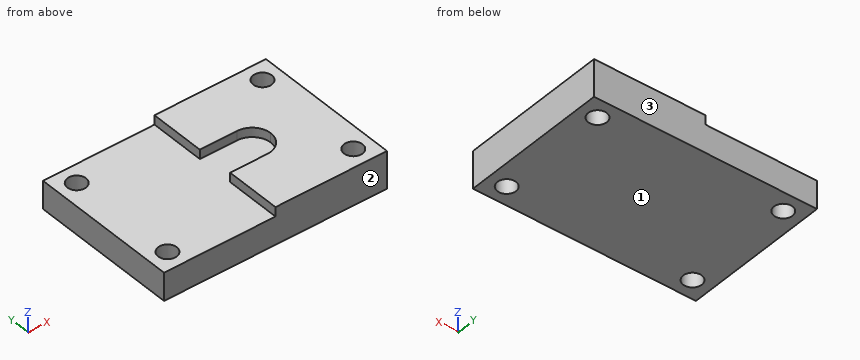
```python
from build123d import *

# Parameters (mm, degrees)
F0_W     = 76.2
F0_H     = 50.8
F1_DEPTH = 12.7
F2_R     = 3.175
F3_DEPTH = 12.701
F5_DEPTH = 3.175
F6_W     = 38.1
F6_H     = 50.8
F7_DEPTH = 3.175


with BuildPart() as f1:
    # F0 (on Top) → F1 (new body)
    with BuildSketch(Plane.XY):
        Rectangle(F0_W, F0_H)
    extrude(amount=F1_DEPTH)

    # F2 (on face) → F3 (cut, through all)
    with BuildSketch(Plane.XY.offset(12.7)):
        with Locations((-31.75, 19.05)):
            Circle(F2_R)
        with Locations((31.75, 19.05)):
            Circle(F2_R)
        with Locations((31.75, -19.05)):
            Circle(F2_R)
        with Locations((-31.75, -19.05)):
            Circle(F2_R)
    extrude(amount=-F3_DEPTH, mode=Mode.SUBTRACT)

    # F4 (on face) → F5 (cut)
    with BuildSketch(Plane.XY.offset(12.7)):
        with BuildLine():
            Line((-12.7, -6.35), (12.7, -6.35))
            ThreePointArc((12.7, -6.35), (17.190128, -4.490128), (19.05, 0))
            ThreePointArc((19.05, 0), (17.190128, 4.490128), (12.7, 6.35))
            Line((12.7, 6.35), (-12.7, 6.35))
            ThreePointArc((-12.7, 6.35), (-17.190128, 4.490128), (-19.05, 0))
            ThreePointArc((-19.05, 0), (-17.190128, -4.490128), (-12.7, -6.35))
        make_face()
    extrude(amount=-F5_DEPTH, mode=Mode.SUBTRACT)

    # F6 (on face) → F7 (cut, through all)
    with BuildSketch(Plane.XY.offset(12.7)):
        with Locations((-19.05, 0)):
            Rectangle(F6_W, F6_H)
    extrude(amount=-F7_DEPTH, mode=Mode.SUBTRACT)


solid = f1.part
```
Build history of the part. All positions in model axes, mm. Face numbers are marked on the shaded views. Give positions to 0.01 mm unless a question says otherwise; leave off trailing zeros. Loops run counter-clockwise (first coordinate to the right, second up) from the corner with the lowest first, then second, coordinate; pieces in that order, holes last. Notation, with made-up numbers: (-34, 61.5) -> (-13, 61.5) arc R7 ccw to (-13, 68.5) -> close; hole circle Ø9 at (78, 54). An arc over 180 degrees is marked (long way). One line per question, with ' | ' between items. Start each with the question number.
1) Cut at C-C (z = 4). Give the cut face in (x, y) (3 decimals), plus the area to 3 significant figures.
2) Pin check, flat tips, straight feed: pin 1 (2.5 mm diameter, centred on y = 17, z = 11.5, fed in from -X); pin 2 (4 mm diameter, centred on x = 31.75, y = -19.05, fed in from -Z) (3 decimals). Stop position of each tip, or through.
3) Cut at B-B (x = -31.75). Give the cut face in (y, z) (3 decimals).
4) Probe L1, parallel to Y at x = 2, z = 11; L2, parallel to Y at x = -31.75, z = 5.25 (3 decimals); L3, parallel to Y at x = -29.5, z = 6. List the from-to ranges inside material, lowest first.
5) Two-plate mould, pull along Y, no slides. Class the marked faces 1, 2 and 3: released by +Y, released by -Y, zero draft, split by the parting line, or undercut.
6) Cut at A-A (y = -19.05). Give the cut face in (x, z) (3 decimals).
7) Cut at D-D (y = 14). Give the cut face in (x, z) (3 decimals), plus the area to 3 significant figures.
Return value:
1) outline: (-38.1, -25.4) -> (38.1, -25.4) -> (38.1, 25.4) -> (-38.1, 25.4) -> close; hole circle Ø6.35 at (-31.75, -19.05); hole circle Ø6.35 at (-31.75, 19.05); hole circle Ø6.35 at (31.75, -19.05); hole circle Ø6.35 at (31.75, 19.05) | area: 3,740 mm^2
2) pin 1: x = 0 | pin 2: through
3) outline: (-25.4, 0) -> (-22.225, 0) -> (-22.225, 9.525) -> (-25.4, 9.525) -> close; (-15.875, 0) -> (15.875, 0) -> (15.875, 9.525) -> (-15.875, 9.525) -> close; (22.225, 0) -> (25.4, 0) -> (25.4, 9.525) -> (22.225, 9.525) -> close
4) L1: -25.4 to -6.35, 6.35 to 25.4 | L2: -25.4 to -22.225, -15.875 to 15.875, 22.225 to 25.4 | L3: -25.4 to -21.29, -16.81 to 16.81, 21.29 to 25.4
5) face 1: zero draft | face 2: released by -Y | face 3: released by +Y
6) outline: (-38.1, 0) -> (-34.925, 0) -> (-34.925, 9.525) -> (-38.1, 9.525) -> close; (-28.575, 0) -> (28.575, 0) -> (28.575, 12.7) -> (0, 12.7) -> (0, 9.525) -> (-28.575, 9.525) -> close; (34.925, 0) -> (38.1, 0) -> (38.1, 12.7) -> (34.925, 12.7) -> close
7) outline: (-38.1, 0) -> (38.1, 0) -> (38.1, 12.7) -> (0, 12.7) -> (0, 9.525) -> (-38.1, 9.525) -> close | area: 847 mm^2
